CAD build for the part. Positions are in the model's coordinates, mm. Face numbers are marked on the shaded views. A direction names the side the tool comes from. Give positions to 0.01 mm unless a question says otherwise; leave off trailing zeros. Write each loop counter-clockwise with the first axis right and the second up, starting at its lowest first coordinate (ties: lowest second). Pieces come first, ordered by that corner, then holes. Notation, with made-up numbers: (21.25, 33.5) - (66.25, 33.5) arc R17 cw to (66.25, 49.5) - close; hole circle Ø5 at (54, 34.25). An arc over 180 degrees is marked (long way). Answer as a JSON object with one key per item and string values.
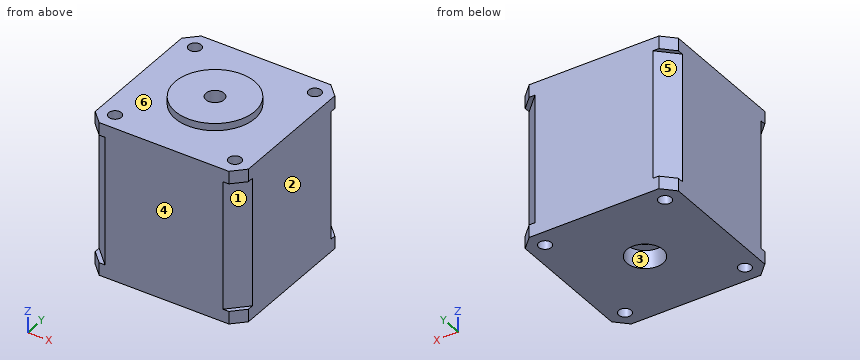
from build123d import *

# Parameters (mm, degrees)
SKETCH1_W                = 42.3
SKETCH1_H                = 42.3
BOSS_EXTRUDE1_DEPTH      = 42.5
SKETCH2_R                = 11
BOSS_EXTRUDE2_DEPTH      = 2
SKETCH3_R                = 1.75
CUT_EXTRUDE1_DEPTH       = 43.5
CUT_EXTRUDE2_DEPTH       = 43.5
SKETCH5_R                = 2.5
CUT_EXTRUDE3_DEPTH       = 45.5
SKETCH6_R                = 2.5
BOSS_EXTRUDE3_DEPTH      = 22
BOSS_EXTRUDE3_DEPTH_BACK = 47.5
SKETCH7_R                = 5
SKETCH7_R_2              = 2.5
CUT_EXTRUDE4_DEPTH       = 5
CUT_EXTRUDE5_DEPTH       = 20
SKETCH9_R                = 2.5
CUT_EXTRUDE6_DEPTH       = 70.5
CUT_EXTRUDE7_DEPTH       = 35.5


with BuildPart() as part:
    # Sketch1 → Boss-Extrude1 (new body)
    with BuildSketch(Plane.XY):
        Rectangle(SKETCH1_W, SKETCH1_H)
    extrude(amount=BOSS_EXTRUDE1_DEPTH)

    # Sketch2 → Boss-Extrude2 (add)
    with BuildSketch(Plane.XY.offset(42.5)):
        Circle(SKETCH2_R)
    extrude(amount=BOSS_EXTRUDE2_DEPTH)

    # Sketch3 → Cut-Extrude1 (cut, through all)
    with BuildSketch(Plane.XY.offset(42.5)):
        with Locations((-16.55, 16.55)):
            Circle(SKETCH3_R)
        with Locations((16.55, 16.55)):
            Circle(SKETCH3_R)
        with Locations((16.55, -16.55)):
            Circle(SKETCH3_R)
        with Locations((-16.55, -16.55)):
            Circle(SKETCH3_R)
    extrude(amount=-CUT_EXTRUDE1_DEPTH, mode=Mode.SUBTRACT)

    # Sketch4 → Cut-Extrude2 (cut, through all)
    with BuildSketch(Plane.XY.offset(42.5)):
        Polygon((-21.15, 17.897308807), (-21.15, 21.15), (-17.897308807, 21.15), align=None)
        Polygon((17.897308807, 21.15), (21.15, 21.15), (21.15, 17.897308807), align=None)
        Polygon((21.15, -17.897308807), (21.15, -21.15), (17.897308807, -21.15), align=None)
        Polygon((-17.897308807, -21.15), (-21.15, -21.15), (-21.15, -17.897308807), align=None)
    extrude(amount=-CUT_EXTRUDE2_DEPTH, mode=Mode.SUBTRACT)

    # Sketch5 → Cut-Extrude3 (cut, through all)
    with BuildSketch(Plane.XY.offset(44.5)):
        Circle(SKETCH5_R)
    extrude(amount=-CUT_EXTRUDE3_DEPTH, mode=Mode.SUBTRACT)

    # Sketch6 → Boss-Extrude3 (add, two sides)
    with BuildSketch(Plane.XY.offset(44.5)) as boss_extrude3_sk:
        Circle(SKETCH6_R)
    extrude(amount=BOSS_EXTRUDE3_DEPTH)
    extrude(boss_extrude3_sk.sketch, amount=-BOSS_EXTRUDE3_DEPTH_BACK)

    # Sketch7 → Cut-Extrude4 (cut)
    with BuildSketch(Plane(origin=(0, 0, 0), x_dir=(-1, 0, 0), z_dir=(0, 0, -1))):
        Circle(SKETCH7_R)
        Circle(SKETCH7_R_2, mode=Mode.SUBTRACT)
    extrude(amount=-CUT_EXTRUDE4_DEPTH, mode=Mode.SUBTRACT)

    # Sketch8 → Cut-Extrude5 (cut)
    with BuildSketch(Plane.XY.offset(66.5)):
        with BuildLine():
            Line((2.5, 0), (0, 2.5))
            ThreePointArc((0, 2.5), (1.767766953, 1.767766953), (2.5, 0))
        make_face()
    extrude(amount=-CUT_EXTRUDE5_DEPTH, mode=Mode.SUBTRACT)

    # Sketch9 → Cut-Extrude6 (cut, through all)
    with BuildSketch(Plane.XY.offset(66.5)):
        Circle(SKETCH9_R)
    extrude(amount=-CUT_EXTRUDE6_DEPTH, mode=Mode.SUBTRACT)

    # Sketch10 → Cut-Extrude7 (cut)
    with BuildSketch(Plane.XY.offset(3.5)):
        Polygon((25, -25), (12.42096321, -25), (25, -12.42096321), align=None)
        Polygon((25, 25), (12.42096321, 25), (25, 12.42096321), align=None)
        Polygon((-25, -25), (-25, -12.42096321), (-12.42096321, -25), align=None)
        Polygon((-25, 12.42096321), (-25, 25), (-12.42096321, 25), align=None)
    extrude(amount=CUT_EXTRUDE7_DEPTH, mode=Mode.SUBTRACT)


solid = part.part
Item 1: Flat gauge pins, fed straight in: P1, Ø3, axis at x = 0, y = 0, coming from the -Z side; P2, Ø4.5, axis at x = 16.55, y = 16.55, coming from the +Z side. Where does each tip first touch, or does it go through?
Entries:
{"P1": "through", "P2": "z = 42.5"}
Item 2: Mould opens along Y. For the marked faces 1, 2 and 3 say: +Y half, -Y half, draft (parallel to the pull), parting line (faces both ways), or undercut.
Entries:
{"face 1": "-Y half", "face 2": "draft", "face 3": "undercut"}
Item 3: Cut at D-D (x = -6). Give the cut face in (y, z), and give its area (3 significant figures).
Entries:
{"outline": "(-21.15, 0) - (21.15, 0) - (21.15, 42.5) - (9.22, 42.5) - (9.22, 44.5) - (-9.22, 44.5) - (-9.22, 42.5) - (-21.15, 42.5) - close", "area": "1,830 mm2"}
Item 4: Probe line 1 (X direction, y = 17, z = 24.5); line 2 (Y direction, x = 0, z = 30); line 3 (Y direction, x = 16.55, z = 14). List the from-to ranges inside material, lowest first. Write a range as from..to.
Entries:
{"line 1": "-20.42..-18.24, -14.86..14.86, 18.24..20.42", "line 2": "-21.15..-2.5, 2.5..21.15", "line 3": "-20.87..-18.3, -14.8..14.8, 18.3..20.87"}
Item 5: Which spindle directions (+Z, -Z, +X, -X, +Y, -Y) get a long thin tool onto all of the face, cutting with end or side? Do the marked faces 4, 5 and 6. Say none if no direction does.
Entries:
{"face 4": "+Z, -Z, +X, -X, -Y", "face 5": "-X, +Y", "face 6": "+Z"}
Item 6: Cut at C-C (z = 20.5). Give the cut face in (x, y).
Entries:
{"outline": "(-21.15, -16.27) - (-16.27, -21.15) - (16.27, -21.15) - (21.15, -16.27) - (21.15, 16.27) - (16.27, 21.15) - (-16.27, 21.15) - (-21.15, 16.27) - close; hole circle Ø3.5 at (-16.55, -16.55); hole circle Ø3.5 at (-16.55, 16.55); hole circle Ø5 at (0, 0); hole circle Ø3.5 at (16.55, -16.55); hole circle Ø3.5 at (16.55, 16.55)"}
Item 7: Cut at A-A (x = 0). Give the cut face in (y, z), and give its area (3 significant figures).
Entries:
{"outline": "(-21.15, 0) - (-5, 0) - (-5, 5) - (-2.5, 5) - (-2.5, 44.5) - (-11, 44.5) - (-11, 42.5) - (-21.15, 42.5) - close; (2.5, 5) - (5, 5) - (5, 0) - (21.15, 0) - (21.15, 42.5) - (11, 42.5) - (11, 44.5) - (2.5, 44.5) - close", "area": "1,590 mm2"}
